Verification items for the finished model (mm, model axes). A direction names the side the tool comes from. Give positions to 0.01 mm unless a question says otherwise; leave off trailing zeros. Loops run counter-clockwise (first coordinate to the right, second up) from the corner with the lowest first, then second, coordinate; pieces in that order, holes last. Notation, with made-up numbers: (-10, -25.75) - (23, -25.75) arc R28 ccw to (23, -4.75) - close; hole circle Ø8 at (5.5, 14.5). An arc over 180 degrees is marked (long way). Use one line per item in the form item = value.
```python
from build123d import *

# Parameters (mm, degrees)
F1_DEPTH = 1.5875
F2_R     = 1.58749


# Not quite as in the source:
# - a fillet or chamfer is up to 0.001 mm smaller than in the source, because OpenCascade refuses the exact size


with BuildPart() as f1:
    # F0 (on Right) → F1 (new body, symmetric)
    with BuildSketch(Plane.YZ):
        with BuildLine():
            Line((6.35, 3.8481), (-6.35, 3.8481))
            Line((-6.35, 3.8481), (-6.35, -3.8481))
            Line((-6.35, -3.8481), (-1.0414, -3.8481))
            Line((-1.0414, -3.8481), (-1.0414, 0.2159))
            ThreePointArc((-1.0414, 0.2159), (0, 1.2573), (1.0414, 0.2159))
            Line((1.0414, 0.2159), (1.0414, -3.8481))
            Line((1.0414, -3.8481), (6.35, -3.8481))
            Line((6.35, -3.8481), (6.35, 3.8481))
        make_face()
    extrude(amount=F1_DEPTH, both=True)

    # F2 (radius 1.5875 in the source; OpenCascade refuses exactly that, so slightly less here)
    f2_edges = [f1.edges().sort_by_distance(p)[0] for p in [
        (-1.5875, -6.35, 0),
        (1.5875, -6.35, 0),
        (1.5875, 6.35, 0),
        (-1.5875, 6.35, 0),
    ]]
    fillet(f2_edges, radius=F2_R)


solid = f1.part
```
1. Depth check by flat-ended pin: pin 1 Ø1.5 at (x, z) = (1, -0.5) entering from +Y. Enter the tip coordinate at first touch or a pass-through.
Result set:
pin_1 = 6.33
2. Draft check along Y on faces 1 (the cylindrical face through (1.11, 5.9, 0.05)), 2 (the flat face through (1.588, -1, 1)), 3 (the flat face through (0, 1.041, -2)). Enter one of: released by +Y, released by -Y, zero draft, split by the parting line, or undercut.
Result set:
face_1 = released by +Y
face_2 = zero draft
face_3 = undercut
3. Section check B-B, the plane x = 0.5. Record the cut outline in (y, z).
Result set:
outline = (-6.27, -3.85) - (-1.04, -3.85) - (-1.04, 0.22) arc R1.04 cw to (1.04, 0.22) - (1.04, -3.85) - (6.27, -3.85) - (6.27, 3.85) - (-6.27, 3.85) - close
4. Tool access check on faces 4 (the flat face through (0, -1.041, -2)), 5 (the cylindrical face through (1.135, -5.873, -0.054)). Record the directions out of +Z, -Z, +X, -X, +Y, -Y that give a thin tool (end or side, any length) a straight path to the whole face; none if there is none.
Result set:
face_4 = -Z, +X, -X
face_5 = +Z, -Z, +X, -Y
5. Section check C-C, the plane y = 0. Record the cut outline in (x, z), then the cut area to 3 significant figures.
Result set:
outline = (-1.59, 1.26) - (1.59, 1.26) - (1.59, 3.85) - (-1.59, 3.85) - close
area = 8.23 mm²
6. Scan lines: probe 1 along Y at (x, z) = (0.1, -2.75); probe 2 along Y at (x, z) = (-0.35, 1); probe 3 along Z at (x, y) = (-1.3, -0.75). Record each from-to range of solid material in increasing order.
Result set:
probe_1 = -6.35 to -1.04, 1.04 to 6.35
probe_2 = -6.31 to -0.69, 0.69 to 6.31
probe_3 = 0.94 to 3.85
